Autodesk Inventor part; units mm, degrees
ref_plane "YZ Plane" through (0, 0, 0) normal (1, 0, 0) x (0, 1, 0)
ref_plane "XZ Plane" through (0, 0, 0) normal (0, 1, 0) x (-1, 0, 0)
ref_plane "XY Plane" through (0, 0, 0) normal (0, 0, 1) x (1, 0, 0)
sketch "Sketch1" plane through (0, 0, 0) normal (0, 0, 1) x (1, 0, 0)
  line L0 (-300, 150) -> (300, 150)
  line L1 (300, 150) -> (300, -150)
  line L2 (300, -150) -> (-300, -150)
  line L3 (-300, -150) -> (-300, 150)
  line L4 (-300, 150) -> (-260, 150)
  line L5 (-260, 150) -> (-260, 1103.1848)
  line L6 (-300, 1103.1848) -> (-300, 150)
  line L7 (300, 150) -> (260, 150)
  line L8 (260, 150) -> (260, 890)
  line L9 (260, 890) -> (300, 890)
  line L10 (300, 890) -> (300, 150)
  line L11 (300, 890) -> (560, 890)
  line L12 (560, 890) -> (560, 850)
  line L13 (560, 850) -> (300, 850)
  line L14 (300, 850) -> (300, 890)
  line L15 (-260, 110) -> (260, 110)
  line L16 (260, 110) -> (260, -110)
  line L17 (260, -110) -> (-260, -110)
  line L18 (-260, -110) -> (-260, 110)
  arc A0 (-260, 1103.1848) -> (-595.8135, 1250) centre (-460, 1103.1848) ccw
  arc A1 (-300, 1103.1848) -> (-568.6508, 1220.637) centre (-460, 1103.1848) ccw
  line L19 (-568.6508, 1220.637) -> (-595.8135, 1250)
  line L20 (-300, 1103.1848) -> (-260, 1103.1848)
  point P0 (0, 0)
  point P1 (0, 110)
  point P2 (-260, 0)
  dimension "d0" = 40
  dimension "d1" = 40
  dimension "d2" = 40
  dimension "d3" = 40
  dimension "d4" = 40
  dimension "d6" = 600
  dimension "d7" = 1400
  dimension "d8" = 1000
  dimension "d9" = 300
  dimension "d29" = 200
  dimension "d30" = 300
extrude "Extrusion1" add sketch "Sketch1" along normal mid plane 400
sketch "Sketch2" plane through (-300, -150, 200) normal (0, -1, 0) x (1, 0, 0)
  line L0 (40, 0) -> (40, -400)
  line L1 (560, 0) -> (560, -400)
  line L2 (600, -400) -> (600, 0)
  line L3 (0, 0) -> (600, 0)
  line L4 (600, -400) -> (0, -400)
  line L5 (0, -400) -> (0, 0)
  line L6 (-268.6508, 0) -> (0, 0)
  line L7 (0, -400) -> (-268.6508, -400)
  line L8 (-268.6508, -400) -> (-268.6508, 0)
  line L9 (600, 0) -> (860, 0)
  line L10 (860, -400) -> (860, 0)
  line L11 (860, -400) -> (600, -400)
  line L12 (0, -400) -> (0, 0)
  line L13 (-228.6508, -40) -> (0, -40)
  line L14 (0, -40) -> (0, -360)
  line L15 (0, -360) -> (-228.6508, -360)
  line L16 (-228.6508, -360) -> (-228.6508, -40)
  line L17 (560, -400) -> (560, 0)
  line L18 (40, -40) -> (560, -40)
  line L19 (560, -40) -> (560, -360)
  line L20 (560, -360) -> (40, -360)
  line L21 (40, -360) -> (40, -40)
  line L22 (600, -40) -> (820, -40)
  line L23 (820, -40) -> (820, -360)
  line L24 (820, -360) -> (600, -360)
  line L25 (600, -360) -> (600, -40)
  point P0 (300, -200)
  point P1 (-228.6508, -200)
  dimension "d14" = 40
  dimension "d15" = 40
  dimension "d16" = 40
  dimension "d17" = 40
  dimension "d18" = 40
  dimension "d19" = 40
extrude "Extrusion2" cut sketch "Sketch2" against normal through all contours L18 L1 L20 L0 | L5 L15 L16 L13 | L22 L23 L24 L2
sketch "Sketch3" plane through (300, -150, -200) normal (1, 0, 0) x (0, 0, -1)
  line L0 (0, 1000) -> (-400, 1000)
  line L1 (-400, 0) -> (-400, 1000)
  line L2 (0, 1000) -> (0, 0)
  line L3 (0, 0) -> (-400, 0)
  line L4 (-360, 260) -> (-400, 260)
  line L5 (0, 260) -> (-40, 260)
  line L6 (-400, 40) -> (-360, 40)
  line L7 (-40, 40) -> (0, 40)
  line L8 (0, 1040) -> (-400, 1040)
  line L9 (-40, 1373.1848) -> (-360, 1373.1848)
  line L10 (-40, 1397.7084) -> (-360, 1397.7084)
  line L11 (-360, 260) -> (-40, 260)
  line L12 (-40, 260) -> (-40, 40)
  line L13 (-40, 40) -> (-360, 40)
  line L14 (-360, 40) -> (-360, 260)
  line L15 (-360, 300) -> (-400, 300)
  line L16 (-360, 1000) -> (-40, 1000)
  line L17 (-40, 1000) -> (-40, 300)
  line L18 (-40, 300) -> (-360, 300)
  line L19 (-360, 300) -> (-360, 1000)
  line L20 (0, 1040) -> (-400, 1040)
  line L21 (-40, 1373.1848) -> (-40, 1453.1848)
  line L22 (-360, 1040) -> (-40, 1040)
  line L23 (-40, 1040) -> (-40, 1200.2849)
  line L24 (-40, 1200.2849) -> (-360, 1200.2849)
  line L25 (-360, 1200.2849) -> (-360, 1040)
  point P0 (-200, 150)
  point P1 (-200, 260)
  point P2 (-360, 150)
  point P3 (-380, 260)
  point P4 (-200, 300)
  point P5 (-40, 1441.0334)
  dimension "d22" = 40
  dimension "d23" = 40
  dimension "d24" = 160.2849
extrude "Extrusion3" cut sketch "Sketch3" against normal through all contours L17 L18 L19 L0 | L12 L13 L14 L11 | L8 L25 L24 L23
sketch "Sketch4" plane through (-260, 150, -200) normal (1, 0, 0) x (0, 0, -1)
  line L0 (-360, 740) -> (-40, 740)
  line L1 (0, 953.1848) -> (-40, 953.1848)
  line L2 (0, -300) -> (0, 953.1848)
  line L3 (0, -300) -> (-400, -300)
  line L4 (-400, 953.1848) -> (-400, -300)
  line L5 (-360, -40) -> (-360, -260)
  line L6 (-360, -260) -> (-40, -260)
  line L7 (-40, -260) -> (-40, -40)
  line L8 (-40, -40) -> (-360, -40)
  line L9 (-360, 700) -> (-360, 0)
  line L10 (-360, 0) -> (-40, 0)
  line L11 (-40, 0) -> (-40, 700)
  line L12 (-40, 700) -> (-360, 700)
  line L13 (-360, 0) -> (-360, 700)
  line L14 (-400, 953.1848) -> (0, 953.1848)
  line L15 (-360, 700) -> (-40, 700)
  line L16 (-40, 700) -> (-40, 876.7461)
  line L17 (-40, 876.7461) -> (-360, 876.7461)
  line L18 (-360, 876.7461) -> (-360, 700)
  line L19 (-40, 740) -> (-40, 900.2849)
  line L20 (-40, 900.2849) -> (-360, 900.2849)
  line L21 (-360, 900.2849) -> (-360, 740)
  line L22 (-360, 953.1848) -> (-360, 1073.1848)
  line L23 (-40, 1073.1848) -> (-360, 1073.1848)
  line L24 (-40, 953.1848) -> (-40, 1073.1848)
  line L25 (-360, 953.1848) -> (-400, 953.1848)
  point P0 (-200, -150)
extrude "Extrusion4" cut sketch "Sketch4" against normal up to next contours L18 L17 L16 L0 | L0 L16 L12 L18
properties part number "Frame"
Verification items for the finished model (mm, model axes). A direction names the side the tool comes from. Coordinates: 2 decimals unless noted, no trailing zeros. Loops run counter-clockwise (first coordinate to the right, second up) from the corner with the lowest first, then second, coordinate; pieces in that order, holes last. Notation, with made-up numbers: (-23, 15.5) - (28, 15.5) arc R14 cw to (28, 25.5) - close; hole circle Ø11 at (-2.5, 38.5). An arc over 180 degrees is marked (long way). Return JSON: item names as keys, results as strings.
1. Section check B-B, the plane y = 907.5. Record the boundary of the cut face in (x, z).
Established:
{"outline": "(-300, -200) - (-260, -200) - (-260, -160) - (-300, -160) - close; (-300, 160) - (-260, 160) - (-260, 200) - (-300, 200) - close"}
2. Section check C-C, the plane x = 127. Record the boundary of the cut face in (y, z), then the cut area to 3 significant figures.
Established:
{"outline": "(-150, -200) - (-110, -200) - (-110, -160) - (-150, -160) - close; (-150, 160) - (-110, 160) - (-110, 200) - (-150, 200) - close; (110, -200) - (150, -200) - (150, -160) - (110, -160) - close; (110, 160) - (150, 160) - (150, 200) - (110, 200) - close", "area": "6,400 mm2"}
3. Mould release check, pull along Y, two halves, no side actions. Record for faces 4 (the flat face through (280, -110, -2)), 5 (the flat face through (412, 870, -160)), 6 (the flat face through (541, 890, -3)), 7 (the flat face through (527, 850, 14)): +Y half, -Y half, draft (parallel to the pull), parting line (faces both ways), or undercut.
Established:
{"face 4": "undercut", "face 5": "draft", "face 6": "+Y half", "face 7": "-Y half"}
4. Section check A-A, the plane z = 17. Count the separate pieces of the cut face and the enclosed holes in it, then the cut area to 3 significant figures.
Established:
{"separate pieces": "8", "enclosed holes": "0", "area": "17,500 mm2"}
5. Go/stop test with flat-tipped pins: pin 1 (12 mm diameter, centred on y = -138.5, z = -66.5, fed in from +X); pin 2 (3 mm diameter, centred on y = 1080, z = -60, fed in from -X); pin 3 (20 mm diameter, centred on x = 283.5, z = -41, fed in from +Y). Record where each tip stops, or that it passes through.
Established:
{"pin 1": "stops at x = 300", "pin 2": "stops at x = -300", "pin 3": "stops at y = 890"}
6. Tool access check on faces 1 (the flat face through (-280, 1050.285, -2)), 2 (the flat face through (-260, -2, 180)), 3 (the flat face through (-260, 130, 2)). Record the directions out of +Z, -Z, +X, -X, +Y, -Y that give a thin tool (end or side, any length) a straight path to the whole face; none if there is none.
Established:
{"face 1": "+X, -X", "face 2": "+Z, -Z", "face 3": "+Y, -Y"}
7. Section check D-D, the plane y = 230.5. Record the boundary of the cut face in (x, z), then the cut area to 3 significant figures.
Established:
{"outline": "(-300, -200) - (-260, -200) - (-260, -160) - (-300, -160) - close; (-300, 160) - (-260, 160) - (-260, 200) - (-300, 200) - close; (260, -200) - (300, -200) - (300, -160) - (260, -160) - close; (260, 160) - (300, 160) - (300, 200) - (260, 200) - close", "area": "6,400 mm2"}
8. Thickness scan on L1, parallel to X at y = 75, z = -171; L2, parallel to X at y = 864, z = 21.5; L3, parallel to Z at x = 268, y = 287. Record the ranges inside material, lowest first.
Established:
{"L1": "x = -300 to -260, 260 to 300", "L2": "x = 260 to 300, 520 to 560", "L3": "z = -200 to -160, 160 to 200"}
